from build123d import *

# Parameters (mm, degrees)
F1_DEPTH      = 9.525
F1_DEPTH_BACK = 9.525
F3_D          = 7.1374


with BuildPart() as f1:
    # F0 (on Front) → F1 (new body, two sides)
    with BuildSketch(Plane.XZ) as f1_sk:
        with BuildLine():
            Line((-762, 11.6416666667), (-762, 0))
            Line((-762, 0), (762, 0))
            Line((762, 0), (762, 11.6416666667))
            ThreePointArc((762, 11.6416666667), (702.4840979371, 155.3257646038), (558.8, 214.8416666667))
            Line((558.8, 214.8416666667), (-558.8, 214.8416666667))
            ThreePointArc((-558.8, 214.8416666667), (-702.4840979371, 155.3257646038), (-762, 11.6416666667))
        make_face()
    extrude(amount=F1_DEPTH)
    extrude(f1_sk.sketch, amount=-F1_DEPTH_BACK)

    # F3 (through all)
    with Locations(Plane.XZ.offset(9.525)):
        with Locations((-406.4, 25.4), (406.4, 25.4)):
            Hole(F3_D / 2)


solid = f1.part
CAD build for the part. Positions are in the model's coordinates, mm. Coordinates: 2 decimals unless noted, no trailing zeros. Write each loop counter-clockwise with the first axis right and the second up, starting at its lowest first coordinate (ties: lowest second). Pieces come first, ordered by that corner, then holes. Notation, with made-up numbers: (-5.75, 45) - (12.25, 45) arc R8 ccw to (12.25, 56) - close; hole circle Ø1 at (-17.75, 26). An arc over 180 degrees is marked (long way). Use a Markdown table: item, result. Add a question column.
Item 1: Band-saw the part on B-B, the plane z = 181. Give the cut face in (x, y) (3 decimals).
Item 2: Band-saw the part on C-C, the plane z = 126. Give the cut face in (x, y) (1 decimal).
Item 3: Drill centre lines: L1, parallel to Z at x = 406.4, y = 2.75; L2, parallel to X at y = 3.5, z = 104; L3, parallel to X at y = -2.25, z = 55.5. Where is each one in solid material? Low to high. Write a range as from..to.
Item 4: Flat gauge pins, fed straight in: pin 1 (6 mm diameter, centred on y = -2.5, z = 145, fed in from +X); pin 2 (6 mm diameter, centred on y = -6.5, z = 176, fed in from -X); pin 3 (4.5 mm diameter, centred on x = 406.4, z = 25.4, fed in from -Y); pin 4 (3 mm diameter, centred on y = -4, z = 140, fed in from -X). Where does each tip first touch, or does it go through?
Item 5: Band-saw the part on A-A, the plane y = 1. Give the cut face in (x, z).
Numbers:
| question | item | result |
|---|---|---|
| 1 | outline | (-671.085, -9.525) - (671.085, -9.525) - (671.085, 9.525) - (-671.085, 9.525) - close |
| 2 | outline | (-726.8, -9.5) - (726.8, -9.5) - (726.8, 9.5) - (-726.8, 9.5) - close |
| 3 | L1 | 0..21.83, 28.97..214.84 |
| 3 | L2 | -739.8..739.8 |
| 3 | L3 | -757.21..757.21 |
| 4 | pin 1 | x = 714.67 |
| 4 | pin 2 | x = -682.31 |
| 4 | pin 3 | through |
| 4 | pin 4 | x = -717.54 |
| 5 | outline | (-762, 0) - (762, 0) - (762, 11.64) arc R203.2 ccw to (558.8, 214.84) - (-558.8, 214.84) arc R203.2 ccw to (-762, 11.64) - close; hole circle Ø7.14 at (-406.4, 25.4); hole circle Ø7.14 at (406.4, 25.4) |
